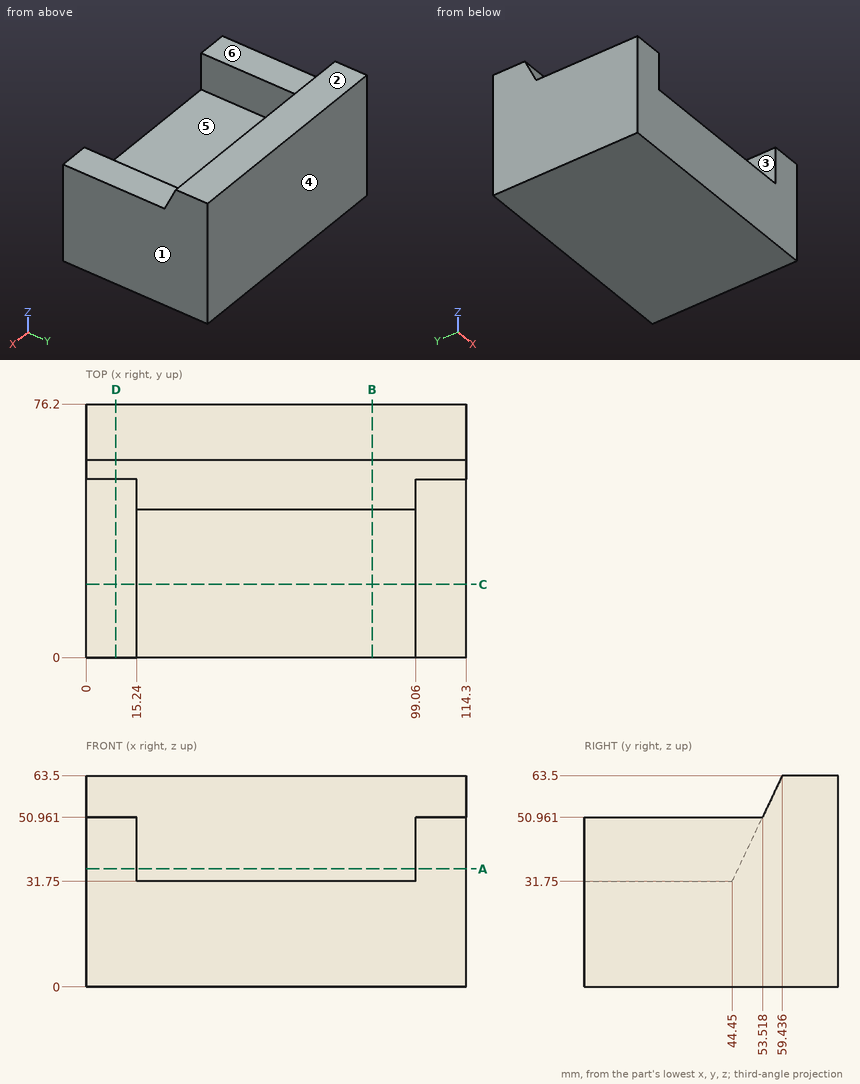
For this review, use the dimensioned drawing (mm, ordinates from the lowest corner) and the shaded views. A direction names the side the tool comes from. Round coordinates to 2 decimals unless told otherwise and drop trailing zeros. Write each loop counter-clockwise with the first axis right and the second up, starting at its lowest first coordinate (ties: lowest second). Pieces come first, ordered by that corner, then holes. Notation, with made-up numbers: (63.5, 86) -> (83.5, 86) arc R24 cw to (83.5, 109) -> close; hole circle Ø5 at (22.25, -17.5). An arc over 180 degrees is marked (long way). One line per item, written item: value. Start each with the question number.
Q1. The part is to be moulded in two halves that separate along X. For the marked faces 1, 2 and 3, say which applies: pulls with the +X half, pulls with the -X half, needs draft (parallel to the pull), parting line crosses it, or undercut.
Q2. Insertion check: P1, Ø22, axis at x = 63, y = 11, coming from the +Z side; P2, Ø7.5, axis at x = 107, y = 13.5, coming from the +Z side. Each pin has a flat end and moves straight along its axis. Give the tip position at first contact, or say it passes through.
Q3. To check wall thickness, follow probe 1 along Z at (x, y) = (103, 49); probe 2 along X at (y, z) = (15, 38); probe 3 along Z at (x, y) = (85, 16). State the ranges of each line that lie inside material, in increasing order.
Q4. Add section B-B (x = 86). Give the boundary of the cut face in (y, z).
Q5. Add section D-D (x = 9). Give the boundary of the cut face in (y, z).
Q6. Tool access review of the marked faces 4, 5 and 6: name each direction out of +Z, -Z, +X, -X, +Y, -Y from which nothing blocks a thin tool from reaching the whole face with its end or side.
Q7. Add section C-C (y = 22). Give the boundary of the cut face in (x, z), then the cut area to 3 significant figures.
Q8. Add section A-A (z = 35.5). Give the boundary of the cut face in (x, y).
Response:
1. face 1: pulls with the +X half
1. face 2: needs draft
1. face 3: undercut
2. P1: stops at z = 31.75
2. P2: stops at z = 50.96
3. probe 1: z = 0 to 50.96
3. probe 2: x = 0 to 15.24, 99.06 to 114.3
3. probe 3: z = 0 to 31.75
4. outline: (0, 0) -> (76.2, 0) -> (76.2, 63.5) -> (59.44, 63.5) -> (44.45, 31.75) -> (0, 31.75) -> close
5. outline: (0, 0) -> (76.2, 0) -> (76.2, 63.5) -> (59.44, 63.5) -> (53.52, 50.96) -> (0, 50.96) -> close
6. face 4: +Z, -Z, +X, -X, +Y
6. face 5: +Z, -Y
6. face 6: +Z, +X, -X, -Y
7. outline: (0, 0) -> (114.3, 0) -> (114.3, 50.96) -> (99.06, 50.96) -> (99.06, 31.75) -> (15.24, 31.75) -> (15.24, 50.96) -> (0, 50.96) -> close
7. area: 4,210 mm^2
8. outline: (0, 0) -> (15.24, 0) -> (15.24, 46.22) -> (99.06, 46.22) -> (99.06, 0) -> (114.3, 0) -> (114.3, 76.2) -> (0, 76.2) -> close
